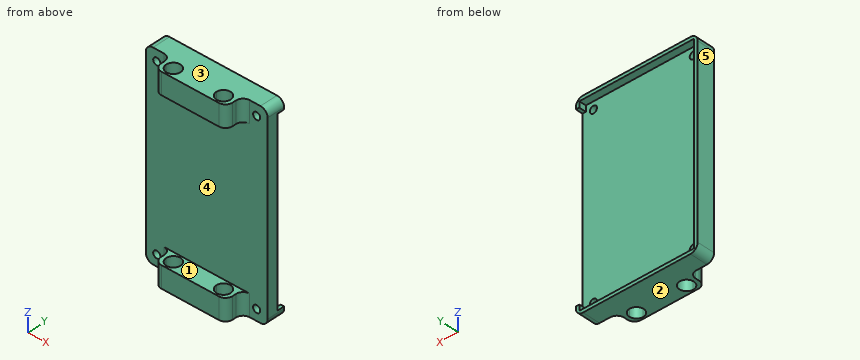
from build123d import *

# Parameters (mm, degrees)
SKETCH_1_W          = 34
SKETCH_1_H          = 55.14
EXTRUDE_1_DEPTH     = 5
SKETCH_2_W          = 32.1
SKETCH_2_H          = 53.24
CUT_EXTRUDE_1_DEPTH = 2
SKETCH_3_W          = 50
SKETCH_3_H          = 10
CUT_EXTRUDE_2_DEPTH = 2
FILLET_3_R          = 2
FILLET_4_R          = 2
FILLET_5_R          = 2
FILLET_6_R          = 2
SKETCH_5_R          = 1
CUT_EXTRUDE_3_DEPTH = 5
CUT_EXTRUDE_5_DEPTH = 5
SKETCH_7_W          = 24.577640881
SKETCH_7_H          = 46.089683544
EXTRUDE_3_DEPTH     = 3
SKETCH_8_W          = 20
SKETCH_8_H          = 6
EXTRUDE_5_DEPTH     = 5
SKETCH_9_W          = 20
SKETCH_9_H          = 6
EXTRUDE_6_DEPTH     = 5
CUT_EXTRUDE_6_DEPTH = 65.972452624
FILLET_7_R          = 2
FILLET_8_R          = 2
FILLET_9_R          = 2
FILLET_10_R         = 2
FILLET_11_R         = 2
FILLET_12_R         = 2
FILLET_13_R         = 2
FILLET_14_R         = 2
SKETCH_11_W         = 2
SKETCH_11_H         = 50
EXTRUDE_7_DEPTH     = 3


with BuildPart() as part:
    # 草图1 → 凸台-拉伸1 (new body)
    with BuildSketch(Plane(origin=(0, 0, 0), x_dir=(1, 0, 0), z_dir=(0, 1, 0))):
        with Locations((17, 27.57)):
            Rectangle(SKETCH_1_W, SKETCH_1_H)
    extrude(amount=EXTRUDE_1_DEPTH)

    # 草图2 → 切除-拉伸1 (cut)
    with BuildSketch(Plane(origin=(0, 5, 0), x_dir=(1, 0, 0), z_dir=(0, 1, 0))):
        with Locations((17, 27.57)):
            Rectangle(SKETCH_2_W, SKETCH_2_H)
    extrude(amount=-CUT_EXTRUDE_1_DEPTH, mode=Mode.SUBTRACT)

    # 草图3 → 切除-拉伸2 (cut)
    with BuildSketch(Plane(origin=(34, 0, 0), x_dir=(0, 0, -1), z_dir=(1, 0, 0))):
        with Locations((27.57, 5)):
            Rectangle(SKETCH_3_W, SKETCH_3_H)
    extrude(amount=-CUT_EXTRUDE_2_DEPTH, mode=Mode.SUBTRACT)

    # 圆角3
    fillet_3_edges = [part.edges().sort_by_distance(p)[0] for p in [
        (0, 2.5, 0),
    ]]
    fillet(fillet_3_edges, radius=FILLET_3_R)

    # 圆角4
    fillet_4_edges = [part.edges().sort_by_distance(p)[0] for p in [
        (0, 2.5, -55.14),
    ]]
    fillet(fillet_4_edges, radius=FILLET_4_R)

    # 圆角5
    fillet_5_edges = [part.edges().sort_by_distance(p)[0] for p in [
        (34, 2.5, -55.14),
    ]]
    fillet(fillet_5_edges, radius=FILLET_5_R)

    # 圆角6
    fillet_6_edges = [part.edges().sort_by_distance(p)[0] for p in [
        (34, 2.5, 0),
    ]]
    fillet(fillet_6_edges, radius=FILLET_6_R)

    # 草图5 → 切除-拉伸3 (cut)
    with BuildSketch(Plane(origin=(0, 3, 0), x_dir=(1, 0, 0), z_dir=(0, 1, 0))):
        with Locations(Location((3.05, 52.09, 0), (0, 0, 270))):
            Circle(SKETCH_5_R)
        with Locations(Location((3.05, 3.05, 0), (0, 0, 90))):
            Circle(SKETCH_5_R)
        with Locations(Location((30.95, 3.05, 0), (0, 0, 270))):
            Circle(SKETCH_5_R)
        with Locations(Location((30.95, 52.09, 0), (0, 0, 90))):
            Circle(SKETCH_5_R)
    extrude(amount=-CUT_EXTRUDE_3_DEPTH, mode=Mode.SUBTRACT)

    # 草图6 → 切除-拉伸5 (cut)
    with BuildSketch(Plane(origin=(0, 3, 0), x_dir=(1, 0, 0), z_dir=(0, 1, 0))):
        with BuildLine():
            ThreePointArc((5.05, 49.09), (5.342893219, 49.797106781), (6.05, 50.09))
            Line((6.05, 50.09), (6.254717451, 50.09))
            ThreePointArc((6.254717451, 50.09), (6.961824232, 49.797106781), (7.254717451, 49.09))
            Line((7.254717451, 49.09), (7.254717451, 6.05))
            ThreePointArc((7.254717451, 6.05), (6.961824232, 5.342893219), (6.254717451, 5.05))
            Line((6.254717451, 5.05), (6.05, 5.05))
            ThreePointArc((6.05, 5.05), (5.342893219, 5.342893219), (5.05, 6.05))
            Line((5.05, 6.05), (5.05, 49.09))
        make_face()
        with BuildLine():
            ThreePointArc((10.05, 49.09), (10.342893219, 49.797106781), (11.05, 50.09))
            Line((11.05, 50.09), (11.254717451, 50.09))
            ThreePointArc((11.254717451, 50.09), (11.961824232, 49.797106781), (12.254717451, 49.09))
            Line((12.254717451, 49.09), (12.254717451, 6.05))
            ThreePointArc((12.254717451, 6.05), (11.961824232, 5.342893219), (11.254717451, 5.05))
            Line((11.254717451, 5.05), (11.05, 5.05))
            ThreePointArc((11.05, 5.05), (10.342893219, 5.342893219), (10.05, 6.05))
            Line((10.05, 6.05), (10.05, 49.09))
        make_face()
        with BuildLine():
            ThreePointArc((20.05, 49.09), (20.342893219, 49.797106781), (21.05, 50.09))
            Line((21.05, 50.09), (21.254717451, 50.09))
            ThreePointArc((21.254717451, 50.09), (21.961824232, 49.797106781), (22.254717451, 49.09))
            Line((22.254717451, 49.09), (22.254717451, 6.05))
            ThreePointArc((22.254717451, 6.05), (21.961824232, 5.342893219), (21.254717451, 5.05))
            Line((21.254717451, 5.05), (21.05, 5.05))
            ThreePointArc((21.05, 5.05), (20.342893219, 5.342893219), (20.05, 6.05))
            Line((20.05, 6.05), (20.05, 49.09))
        make_face()
        with BuildLine():
            ThreePointArc((26.05, 5.05), (25.342893219, 5.342893219), (25.05, 6.05))
            Line((25.05, 6.05), (25.05, 49.09))
            ThreePointArc((25.05, 49.09), (25.342893219, 49.797106781), (26.05, 50.09))
            Line((26.05, 50.09), (26.254717451, 50.09))
            ThreePointArc((26.254717451, 50.09), (26.961824232, 49.797106781), (27.254717451, 49.09))
            Line((27.254717451, 49.09), (27.254717451, 6.05))
            ThreePointArc((27.254717451, 6.05), (26.961824232, 5.342893219), (26.254717451, 5.05))
            Line((26.254717451, 5.05), (26.05, 5.05))
        make_face()
        with BuildLine():
            Line((15.05, 49.09), (15.05, 6.05))
            ThreePointArc((15.05, 6.05), (15.342893219, 5.342893219), (16.05, 5.05))
            Line((16.05, 5.05), (16.254717451, 5.05))
            ThreePointArc((16.254717451, 5.05), (16.961824232, 5.342893219), (17.254717451, 6.05))
            Line((17.254717451, 6.05), (17.254717451, 49.09))
            ThreePointArc((17.254717451, 49.09), (16.961824232, 49.797106781), (16.254717451, 50.09))
            Line((16.254717451, 50.09), (16.05, 50.09))
            ThreePointArc((16.05, 50.09), (15.342893219, 49.797106781), (15.05, 49.09))
        make_face()
    extrude(amount=-CUT_EXTRUDE_5_DEPTH, mode=Mode.SUBTRACT)

    # 草图7 → 凸台-拉伸3 (add)
    with BuildSketch(Plane.XZ):
        with Locations((15.625766317, -27.57)):
            Rectangle(SKETCH_7_W, SKETCH_7_H)
    extrude(amount=-EXTRUDE_3_DEPTH)

    # 草图8 → 凸台-拉伸5 (add)
    with BuildSketch(Plane.XZ):
        with Locations((17, -3)):
            Rectangle(SKETCH_8_W, SKETCH_8_H)
    extrude(amount=EXTRUDE_5_DEPTH)

    # 草图9 → 凸台-拉伸6 (add)
    with BuildSketch(Plane.XZ):
        with Locations((17, -52.14)):
            Rectangle(SKETCH_9_W, SKETCH_9_H)
    extrude(amount=EXTRUDE_6_DEPTH)

    # 草图10 → 切除-拉伸6 (cut, through all)
    with BuildSketch(Plane(origin=(0, 0, -55.14), x_dir=(-1, 0, 0), z_dir=(0, 0, -1))):
        with BuildLine():
            ThreePointArc((-8, -2.5), (-11.414213562, -1.085786438), (-10, -4.5))
            Line((-10, -4.5), (-10, -2.5))
            Line((-10, -2.5), (-8, -2.5))
        make_face()
        with BuildLine():
            Line((-10, -2.5), (-10, -4.5))
            ThreePointArc((-10, -4.5), (-8.585786438, -3.914213562), (-8, -2.5))
            Line((-8, -2.5), (-10, -2.5))
        make_face()
        with BuildLine():
            ThreePointArc((-26, -2.5), (-25.414213562, -3.914213562), (-24, -4.5))
            Line((-24, -4.5), (-24, -2.5))
            Line((-24, -2.5), (-26, -2.5))
        make_face()
        with BuildLine():
            Line((-24, -2.5), (-24, -4.5))
            ThreePointArc((-24, -4.5), (-22.585786438, -3.914213562), (-22, -2.5))
            ThreePointArc((-22, -2.5), (-24, -0.5), (-26, -2.5))
            Line((-26, -2.5), (-24, -2.5))
        make_face()
    extrude(amount=-CUT_EXTRUDE_6_DEPTH, mode=Mode.SUBTRACT)

    # 圆角7
    fillet_7_edges = [part.edges().sort_by_distance(p)[0] for p in [
        (7, -5, -52.14),
    ]]
    fillet(fillet_7_edges, radius=FILLET_7_R)

    # 圆角8
    fillet_8_edges = [part.edges().sort_by_distance(p)[0] for p in [
        (7, 0, -52.14),
    ]]
    fillet(fillet_8_edges, radius=FILLET_8_R)

    # 圆角9
    fillet_9_edges = [part.edges().sort_by_distance(p)[0] for p in [
        (27, -5, -52.14),
    ]]
    fillet(fillet_9_edges, radius=FILLET_9_R)

    # 圆角10
    fillet_10_edges = [part.edges().sort_by_distance(p)[0] for p in [
        (27, 0, -52.14),
    ]]
    fillet(fillet_10_edges, radius=FILLET_10_R)

    # 圆角11
    fillet_11_edges = [part.edges().sort_by_distance(p)[0] for p in [
        (7, -5, -3),
    ]]
    fillet(fillet_11_edges, radius=FILLET_11_R)

    # 圆角12
    fillet_12_edges = [part.edges().sort_by_distance(p)[0] for p in [
        (7, 0, -3),
    ]]
    fillet(fillet_12_edges, radius=FILLET_12_R)

    # 圆角13
    fillet_13_edges = [part.edges().sort_by_distance(p)[0] for p in [
        (27, -5, -3),
    ]]
    fillet(fillet_13_edges, radius=FILLET_13_R)

    # 圆角14
    fillet_14_edges = [part.edges().sort_by_distance(p)[0] for p in [
        (27, 0, -3),
    ]]
    fillet(fillet_14_edges, radius=FILLET_14_R)

    # 草图11 → 凸台-拉伸7 (add)
    with BuildSketch(Plane.XZ):
        with Locations((33, -27.57)):
            Rectangle(SKETCH_11_W, SKETCH_11_H)
    extrude(amount=-EXTRUDE_7_DEPTH)


solid = part.part
Verification items for the finished model (mm, model axes). Face numbers are marked on the shaded views. A direction names the side the tool comes from. Round coordinates to 2 decimals unless told otherwise and drop trailing zeros. Loops run counter-clockwise (first coordinate to the right, second up) from the corner with the lowest first, then second, coordinate; pieces in that order, holes last. Notation, with made-up numbers: (4.25, 81.25) - (28.25, 81.25) arc R10 cw to (28.25, 90.25) - close; hole circle Ø5 at (7, 51.5). An arc over 180 degrees is marked (long way). Answer in a Markdown table with one row per item. Add a question column.
Q1. Section check A-A on x = 30.95. Enter the section's corners in (y, z).
Q2. Tool access check on the marked faces 1 and 2. Record the directions out of +Z, -Z, +X, -X, +Y, -Y that give a thin tool (end or side, any length) a straight path to the whole face; none if there is none.
Q3. Section check C-C on z = -42. Enter the section's corners in (x, y), plus the area to 3 significant figures.
Q4. Material ranges on line 1 (X direction, y = 0.9, z = -3.05); line 2 (Z direction, x = 5, y = 4.5); line 3 (X direction, y = -2.5, z = -51.55), recorded low to high.
Q5. Section check B-B on y = 4. Enter the section's corners in (x, z).
Q6. Section check D-D on x = 21. Enter the section's corners in (y, z), plus the area to 3 significant figures.
Q7. Release check for a two-part mould opening along Z. For the marked faces 3, 4 and 5 record: pulls with the +Z half, pulls with the -Z half, needs draft (parallel to the pull), parting line crosses it, or undercut.
Q8. Gauge pin test, flat ends, axial feed: pin 1 (3 mm diameter, centred on x = 27.5, z = -44, fed in from +Y); pin 2 (0.8 mm diameter, centred on y = -2.5, z = -3.5, fed in from -X); pin 3 (0.6 mm diameter, centred on y = 3.5, z = -23.5, fed in from +X). Record the tip position at first contact, or that the pin passes through.
Found:
| question | item | result |
|---|---|---|
| 1 | outline | (0, -55.14) - (5, -55.14) - (5, -54.19) - (3, -54.19) - (3, -53.09) - (0, -53.09) - close; (0, -51.09) - (3, -51.09) - (3, -4.05) - (0, -4.05) - close; (0, -2.05) - (3, -2.05) - (3, -0.95) - (5, -0.95) - (5, 0) - (0, 0) - close |
| 2 | face 1 | +X, -X, -Y |
| 2 | face 2 | -Z, +X, -X, +Y, -Y |
| 3 | outline | (0, 0) - (34, 0) - (34, 3) - (0.95, 3) - (0.95, 5) - (0, 5) - close |
| 3 | area | 104 mm² |
| 4 | line 1 | x = 0 to 2.05, 4.05 to 29.95, 31.95 to 34 |
| 4 | line 2 | z = -55.14 to -54.19, -0.95 to 0 |
| 4 | line 3 | x = 7 to 8, 12 to 22, 26 to 27 |
| 5 | outline | (0, -53.14) arc R2 ccw to (2, -55.14) - (32, -55.14) arc R2 ccw to (34, -53.14) - (34, -52.57) - (33.05, -52.57) - (33.05, -54.19) - (0.95, -54.19) - (0.95, -0.95) - (33.05, -0.95) - (33.05, -2.57) - (34, -2.57) - (34, -2) arc R2 ccw to (32, 0) - (2, 0) arc R2 ccw to (0, -2) - close |
| 6 | outline | (-5, -55.14) - (5, -55.14) - (5, -54.19) - (3, -54.19) - (3, -0.95) - (5, -0.95) - (5, 0) - (-5, 0) - (-5, -6) - (0, -6) - (0, -49.14) - (-5, -49.14) - close |
| 6 | area | 229 mm² |
| 7 | face 3 | pulls with the +Z half |
| 7 | face 4 | undercut |
| 7 | face 5 | needs draft |
| 8 | pin 1 | stops at y = 3 |
| 8 | pin 2 | stops at x = 7 |
| 8 | pin 3 | stops at x = 0.95 |
